```python
from build123d import *

# Parameters (mm, degrees)
SKETCH1_R           = 3.1
BOSS_EXTRUDE1_DEPTH = 15
SKETCH2_R           = 9.5
CUT_EXTRUDE1_DEPTH  = 1.8
CHAMFER2_SIZE       = 1


with BuildPart() as part:
    # Sketch1 → Boss-Extrude1 (new body)
    with BuildSketch(Plane(origin=(0, 0, 0), x_dir=(1, 0, 0), z_dir=(0, 1, 0))):
        with BuildLine():
            Line((-120, 11), (120, 11))
            ThreePointArc((120, 11), (131, 0), (120, -11))
            Line((120, -11), (-120, -11))
            ThreePointArc((-120, -11), (-131, 0), (-120, 11))
        make_face()
        with Locations(Location((-120, 0, 0), (0, 0, 270))):
            Circle(SKETCH1_R, mode=Mode.SUBTRACT)
        with Locations(Location((120, 0, 0), (0, 0, 270))):
            Circle(SKETCH1_R, mode=Mode.SUBTRACT)
        with Locations(Location((0, 0, 0), (0, 0, 270))):
            Circle(SKETCH1_R, mode=Mode.SUBTRACT)
    extrude(amount=BOSS_EXTRUDE1_DEPTH)

    # Sketch2 → Cut-Extrude1 (cut)
    with BuildSketch(Plane(origin=(0, 15, 0), x_dir=(1, 0, 0), z_dir=(0, 1, 0))):
        with Locations(Location((120, 0, 0), (0, 0, 270))):
            Circle(SKETCH2_R)
        with Locations(Location((0, 0, 0), (0, 0, 270))):
            Circle(SKETCH2_R)
        with Locations(Location((-120, 0, 0), (0, 0, 270))):
            Circle(SKETCH2_R)
    cut_extrude1 = extrude(amount=-CUT_EXTRUDE1_DEPTH, mode=Mode.SUBTRACT)

    # Chamfer2
    chamfer2_edges = [part.edges().sort_by_distance(p)[0] for p in [
        (131, 15, 0),
        (0, 15, -11),
        (-131, 15, 0),
        (0, 0, -11),
        (131, 0, 0),
        (0, 0, 11),
        (-131, 0, 0),
        (0, 15, 11),
    ]]
    chamfer(chamfer2_edges, length=CHAMFER2_SIZE)

    # Mirror1: Cut-Extrude1 across plane
    add(cut_extrude1.mirror(Plane.ZX.offset(7.5)), mode=Mode.SUBTRACT)

    # Chamfer1: read off the stored shape, not the designer's step
    # Chamfer1: loft between two sections, ruled curve by curve
    chamfer1_from = [
        Edge.make_three_point_arc((120, 1, 9.5), (110.5, 1, 0), (120, 1, -9.5)),
        Edge.make_three_point_arc((120, 1, -9.5), (129.5, 1, 0), (120, 1, 9.5)),
    ]
    chamfer1_to = [
        Edge.make_three_point_arc((120, 0, 10.5), (109.5, 0, 0), (120, 0, -10.5)),
        Edge.make_three_point_arc((120, 0, -10.5), (130.5, 0, 0), (120, 0, 10.5)),
    ]
    chamfer1 = Solid(Shell([*[Face.make_surface_from_curves(chamfer1_from[k], chamfer1_to[k]) for k in range(2)], Face(Wire(chamfer1_from)), Face(Wire(chamfer1_to))]))
    add(chamfer1, mode=Mode.SUBTRACT)

    # Chamfer1 2: loft between two sections, ruled curve by curve
    chamfer1_2_from = [
        Edge.make_three_point_arc((2.896651441, 1, -9.047619048), (9.047619048, 1, 2.896651441), (-2.896651441, 1, 9.047619048)),
        Edge.make_three_point_arc((-2.896651441, 1, 9.047619048), (-9.047619048, 1, -2.896651441), (2.896651441, 1, -9.047619048)),
    ]
    chamfer1_2_to = [
        Edge.make_three_point_arc((3.201562119, 0, -10), (10, 0, 3.201562119), (-3.201562119, 0, 10)),
        Edge.make_three_point_arc((-3.201562119, 0, 10), (-10, 0, -3.201562119), (3.201562119, 0, -10)),
    ]
    chamfer1_2 = Solid(Shell([*[Face.make_surface_from_curves(chamfer1_2_from[k], chamfer1_2_to[k]) for k in range(2)], Face(Wire(chamfer1_2_from)), Face(Wire(chamfer1_2_to))]))
    add(chamfer1_2, mode=Mode.SUBTRACT)

    # Chamfer1 3: loft between two sections, ruled curve by curve
    chamfer1_3_from = [
        Edge.make_three_point_arc((-120, 1, 9.5), (-129.5, 1, 0), (-120, 1, -9.5)),
        Edge.make_three_point_arc((-120, 1, -9.5), (-110.5, 1, 0), (-120, 1, 9.5)),
    ]
    chamfer1_3_to = [
        Edge.make_three_point_arc((-120, 0, 10.5), (-130.5, 0, 0), (-120, 0, -10.5)),
        Edge.make_three_point_arc((-120, 0, -10.5), (-109.5, 0, 0), (-120, 0, 10.5)),
    ]
    chamfer1_3 = Solid(Shell([*[Face.make_surface_from_curves(chamfer1_3_from[k], chamfer1_3_to[k]) for k in range(2)], Face(Wire(chamfer1_3_from)), Face(Wire(chamfer1_3_to))]))
    add(chamfer1_3, mode=Mode.SUBTRACT)

    # Chamfer1 4: loft between two sections, ruled curve by curve
    chamfer1_4_from = [
        Edge.make_three_point_arc((120, 14, 9.5), (129.5, 14, 0), (120, 14, -9.5)),
        Edge.make_three_point_arc((120, 14, -9.5), (110.5, 14, 0), (120, 14, 9.5)),
    ]
    chamfer1_4_to = [
        Edge.make_three_point_arc((120, 15, 10.5), (130.5, 15, 0), (120, 15, -10.5)),
        Edge.make_three_point_arc((120, 15, -10.5), (109.5, 15, 0), (120, 15, 10.5)),
    ]
    chamfer1_4 = Solid(Shell([*[Face.make_surface_from_curves(chamfer1_4_from[k], chamfer1_4_to[k]) for k in range(2)], Face(Wire(chamfer1_4_from)), Face(Wire(chamfer1_4_to))]))
    add(chamfer1_4, mode=Mode.SUBTRACT)

    # Chamfer1 5: loft between two sections, ruled curve by curve
    chamfer1_5_from = [
        Edge.make_three_point_arc((0, 14, 9.5), (9.5, 14, 0), (0, 14, -9.5)),
        Edge.make_three_point_arc((0, 14, -9.5), (-9.5, 14, 0), (0, 14, 9.5)),
    ]
    chamfer1_5_to = [
        Edge.make_three_point_arc((0, 15, 10.5), (10.5, 15, 0), (0, 15, -10.5)),
        Edge.make_three_point_arc((0, 15, -10.5), (-10.5, 15, 0), (0, 15, 10.5)),
    ]
    chamfer1_5 = Solid(Shell([*[Face.make_surface_from_curves(chamfer1_5_from[k], chamfer1_5_to[k]) for k in range(2)], Face(Wire(chamfer1_5_from)), Face(Wire(chamfer1_5_to))]))
    add(chamfer1_5, mode=Mode.SUBTRACT)

    # Chamfer1 6: loft between two sections, ruled curve by curve
    chamfer1_6_from = [
        Edge.make_three_point_arc((-120, 14, 9.5), (-110.5, 14, 0), (-120, 14, -9.5)),
        Edge.make_three_point_arc((-120, 14, -9.5), (-129.5, 14, 0), (-120, 14, 9.5)),
    ]
    chamfer1_6_to = [
        Edge.make_three_point_arc((-120, 15, 10.5), (-109.5, 15, 0), (-120, 15, -10.5)),
        Edge.make_three_point_arc((-120, 15, -10.5), (-130.5, 15, 0), (-120, 15, 10.5)),
    ]
    chamfer1_6 = Solid(Shell([*[Face.make_surface_from_curves(chamfer1_6_from[k], chamfer1_6_to[k]) for k in range(2)], Face(Wire(chamfer1_6_from)), Face(Wire(chamfer1_6_to))]))
    add(chamfer1_6, mode=Mode.SUBTRACT)


solid = part.part
```
For this review, take the finished solid that the model builds, in its own axes (mm). A direction names the side the tool comes from. Round coordinates to 2 decimals unless told otherwise and drop trailing zeros. Loops run counter-clockwise (first coordinate to the right, second up) from the corner with the lowest first, then second, coordinate; pieces in that order, holes last.
(1) We need section A-A (y = 4.25). Give the boundary of the cut face in (x, z).
Returned:
outline: (-120, -11) - (120, -11) arc R11 ccw to (120, 11) - (-120, 11) arc R11 ccw to start; hole circle Ø6.2 at (-120, 0); hole circle Ø6.2 at (0, 0); hole circle Ø6.2 at (120, 0)
(2) Wall thickness on line 1 along X through (y, z) = (13.5, 0.75); line 2 along X through (y, z) = (5.75, 0); line 3 along Z through (x, y) = (-120, 8.5): over which ranges is each line inside the solid? List them lowest first.
Returned:
line 1: x = -130.97 to -129.47, -110.53 to -9.47, 9.47 to 110.53, 129.47 to 130.97
line 2: x = -131 to -123.1, -116.9 to -3.1, 3.1 to 116.9, 123.1 to 131
line 3: z = -11 to -3.1, 3.1 to 11
(3) Mouldability with a two-part tool opening along X and no side actions: class faces 1 (the flat face through (-59, 15, 0)), 2 (the conical face through (130.4, 0.4, -0.2)), 3 (the cylindrical face through (-9.274, 1.394, -2.059)) as released by +X, released by -X, zero draft, split by the parting line, or undercut.
Returned:
face 1: zero draft
face 2: released by +X
face 3: undercut
(4) We need section B-B (z = 0). State how many separate pieces and enclosed holes the cut face has, plus the area to 4 significant figures.
Returned:
separate pieces: 4
enclosed holes: 0
area: 3,505 mm2
(5) Tool access review of faces 4 (the flat face through (-2, 7, -11)), 5 (the flat face through (-120, 13.2, 4)), 6 (the flat face through (0, 1.8, 4)): name each direction out of +Z, -Z, +X, -X, +Y, -Y from which nothing blocks a thin tool from reaching the whole face with its end or side.
Returned:
face 4: -Z, +X, -X, +Y, -Y
face 5: +Y
face 6: -Y
(6) Clearance check with flat-ended pins moving along their axes: P1, Ø9.5, axis at x = -4, z = 4, coming from the +Y side; P2, Ø6, axis at y = 9.5, z = 4.5, coming from the -X side; P3, Ø5.5, axis at x = 116.5, z = -1, coming from the +Y side. State where each tip first meets the part, or that it passes through.
Returned:
P1: stops at y = 14.91
P2: stops at x = -130.9
P3: stops at y = 13.2
